```python
from build123d import *

# Parameters (mm, degrees)
SKETCH1_W           = 17.78
SKETCH1_H           = 19.05
SKETCH1_R           = 3.2639
SKETCH1_W_2         = 27.94
BOSS_EXTRUDE3_DEPTH = 6.35
SKETCH3_W           = 22.86
SKETCH3_H           = 19.05
BOSS_EXTRUDE4_DEPTH = 20.32
SKETCH6_R           = 6.604
CUT_EXTRUDE1_DEPTH  = 20.32
FILLET5_R           = 2.54


with BuildPart() as part:
    # Sketch1 → Boss-Extrude3 (new body)
    with BuildSketch(Plane(origin=(0, 0, 0), x_dir=(1, 0, 0), z_dir=(0, 1, 0))):
        with Locations((-26.491045528, -6.411090754)):
            Rectangle(SKETCH1_W, SKETCH1_H)
        with Locations((-25.221045528, -6.411090754)):
            Circle(SKETCH1_R, mode=Mode.SUBTRACT)
        with Locations((-3.631045528, -6.411090754)):
            Rectangle(SKETCH1_W_2, SKETCH1_H)
        with Locations((19.228954472, -6.411090754)):
            Rectangle(SKETCH1_W, SKETCH1_H)
        with Locations((17.958954472, -6.411090754)):
            Circle(SKETCH1_R, mode=Mode.SUBTRACT)
    extrude(amount=BOSS_EXTRUDE3_DEPTH)

    # Sketch3 → Boss-Extrude4 (add)
    with BuildSketch(Plane(origin=(0, 6.35, 0), x_dir=(1, 0, 0), z_dir=(0, 1, 0))):
        with Locations((-3.631045528, -6.411090754)):
            Rectangle(SKETCH3_W, SKETCH3_H)
    extrude(amount=BOSS_EXTRUDE4_DEPTH)

    # Sketch6 → Cut-Extrude1 (cut)
    with BuildSketch(Plane.XY.offset(15.936090754)):
        with Locations((-3.631045528, 16.51)):
            Circle(SKETCH6_R)
    extrude(amount=-CUT_EXTRUDE1_DEPTH, mode=Mode.SUBTRACT)

    # Fillet5
    fillet5_edges = [part.edges().sort_by_distance(p)[0] for p in [
        (-15.061045528, 6.35, 6.411090754),
        (-35.381045528, 6.35, 6.411090754),
        (28.118954472, 6.35, 6.411090754),
        (7.798954472, 26.67, 6.411090754),
        (-15.061045528, 26.67, 6.411090754),
        (7.798954472, 6.35, 6.411090754),
    ]]
    fillet(fillet5_edges, radius=FILLET5_R)


solid = part.part
```
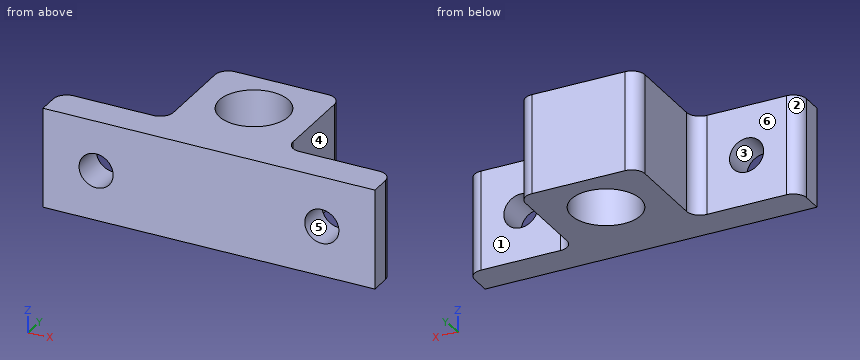
Source: CAD feature listing. Evaluate the final solid. Frame: model axes, mm. Face numbers are marked on the shaded views. A direction names the side the tool comes from. Give positions to 0.01 mm unless a question says otherwise; leave off trailing zeros. Loops run counter-clockwise (first coordinate to the right, second up) from the corner with the lowest first, then second, coordinate; pieces in that order, holes last. Notation, with made-up numbers: (-3.5, 49.25) - (47.5, 49.25) arc R25 ccw to (47.5, 85.25) - close; hole circle Ø3 at (-6, -33.5). An arc over 180 degrees is marked (long way). Use CSV: the item, a comma, the result in double quotes. Start each with the question number.
1. Section B-B (x = 0.5). Output: boundary loops of the cut face in (y, z).
2. Section D-D (x = 24). Output: boundary loops of the cut face in (y, z), then the cut area to 3 significant figures.
3. Section C-C (z = 2.5). Output: boundary loops of the cut face in (x, y).
4. Section A-A (y = 16.51). Output: boundary loops of the cut face in (x, z), then the cut area to 3 significant figures.
5. Draft query along X for the marked faces 1, 2, 3 and 4. Return one class per face: +X half, -X half, draft (parallel to the pull), parting line (faces both ways), or undercut.
6. Ray query, L1, parallel to Y at x = -27, z = -1; L2, parallel to X at y = 16, z = 7.5. Return the intervals inside material, ascending.
7. Reachability of the marked faces 5 and 6 from +Z, -Z, +X, -X, +Y, -Y: full face, straight path, thin tool, end or side. Return the list, or none.
8. Pin query (flat end, axial travel): pin 1 (10 mm diameter, centred on x = -22.5, y = 8, fed in from +Z); pin 2 (4.5 mm diameter, centred on y = 15.5, z = 10, fed in from -X); pin 3 (10.5 mm diameter, centred on x = 17.96, z = 6.41, fed in from +Y); pin 4 (2 mm diameter, centred on y = 9.5, z = 5, fed in from +X). Return the tip coordinate at first contact, or that it passes through.
Response:
1,outline,"(0, -3.11) - (11.36, -3.11) - (11.36, 15.94) - (0, 15.94) - close; (21.66, -3.11) - (26.67, -3.11) - (26.67, 15.94) - (21.66, 15.94) - close"
2,outline,"(0, -3.11) - (6.35, -3.11) - (6.35, 15.94) - (0, 15.94) - close"
2,area,"121 mm²"
3,outline,"(-35.38, 0) - (28.12, 0) - (28.12, 3.81) arc R2.54 ccw to (25.58, 6.35) - (10.34, 6.35) arc R2.54 cw to (7.8, 8.89) - (7.8, 24.13) arc R2.54 ccw to (5.26, 26.67) - (-12.52, 26.67) arc R2.54 ccw to (-15.06, 24.13) - (-15.06, 8.89) arc R2.54 cw to (-17.6, 6.35) - (-32.84, 6.35) arc R2.54 ccw to (-35.38, 3.81) - close; hole circle Ø13.21 at (-3.63, 16.51)"
4,outline,"(-15.06, -3.11) - (-10.24, -3.11) - (-10.24, 15.94) - (-15.06, 15.94) - close; (2.97, -3.11) - (7.8, -3.11) - (7.8, 15.94) - (2.97, 15.94) - close"
4,area,"184 mm²"
5,face 1,"draft"
5,face 2,"-X half"
5,face 3,"undercut"
5,face 4,"+X half"
6,L1,"0 to 6.35"
6,L2,"-15.06 to -10.22, 2.95 to 7.8"
7,face 5,"+Y, -Y"
7,face 6,"+Z, -Z, -X, +Y"
8,pin 1,"z = 15.94"
8,pin 2,"x = -15.06"
8,pin 3,"y = 6.35"
8,pin 4,"x = 7.83"
